Autodesk Inventor part; units mm, degrees
ref_plane "Work Plane1" through (29, 0, 0) normal (0, -1, 0) x (1, 0, 0)
ref_plane "YZ Plane" through (0, 0, 0) normal (1, 0, 0) x (0, 1, 0)
ref_plane "XZ Plane" through (0, 0, 0) normal (0, 1, 0) x (-1, 0, 0)
sketch "Skizze1" plane through (0, 0, 0) normal (0, 0, 1) x (1, 0, 0)
  line L0 (-1.1667, 0) -> (20, 0)
  line L1 (20, 0) -> (20, 2.5)
  line L2 (20, 2.5) -> (2, 2.5)
  line L3 (2, 2.5) -> (1.5091, 2.5)
  line L4 (1.5091, 2.5) -> (0, 2.5)
  line L5 (0, 2.5) -> (0, 4.25)
  line L6 (0, 4.25) -> (-5, 4.25)
  line L7 (-5, 4.25) -> (-5, 2.3094)
  line L8 (-5, 2.3094) -> (-2.5, 2.3094)
  line L9 (-2.5, 2.3094) -> (-1.1667, 0)
  line L10 (-10, 0) -> (25, 0)
  line L11 (0, -0.85) -> (0, 5.1)
  line L12 (2, 2.5) -> (0, 2.5) construction
  dimension "d1" = 18
  dimension "d2" = 0.4909
  dimension "d3" = 5
  dimension "d4" = 2.5
  dimension "d5" = 60
  dimension "d6" = 5
  dimension "d7" = 5
  dimension "d8" = 4.6188
  dimension "d9" = 8.5
  dimension "d26" = 20
revolve "Körper" add sketch "Skizze1" angle 360 about axis through (-1.1667, 0, 0) along (1, 0, 0)
sketch "Skizze2" plane through (-5, 0, 0) normal (-1, 0, 0) x (0, 0, 1)
  circle A0 centre (0, 0) radius 2.3094
  line L0 (0, -5.95) -> (0, 5.95)
  line L1 (-5.95, 0) -> (5.95, 0)
  line L2 (2.3094, 0) -> (1.1547, -2)
  line L3 (1.1547, -2) -> (-1.1547, -2)
  line L4 (-1.1547, -2) -> (-2.3094, 0)
  line L5 (-2.3094, 0) -> (-1.1547, 2)
  line L6 (-1.1547, 2) -> (1.1547, 2)
  line L7 (1.1547, 2) -> (2.3094, 0)
extrude "Loch" add sketch "Skizze2" against normal up to next contours L7 A0 | A0 L2 | L6 L0 A0 | A0 L0 L3 | L0 L6 A0 | A0 L3 L0 | L4 A0 | A0 L5
fillet "Rundung1" radius 0.5 1 edges at (-5, -4.25, 0)
thread "Gewinde"
chamfer "Fase1" distance 0.4908 distance2 0.4908 1 edges at (20, -2.5, 0) measured on face at (20, -0.7379, -0.3873)
ref_plane "Work Plane1" through (29, 0, 0) normal (0, -1, 0) x (1, 0, 0)
fillet "Fillet2" radius 0.1 1 edges at (0, -2.5, 0)
sketch "Skizze4" plane through (0, 0, 0) normal (0, 1, 0) x (-1, 0, 0)
  line L0 (-19.5092, 2.5) -> (-19.5092, -2.5)
  line L1 (-0.1, -2.5) -> (-0.1, 2.5)
  line L2 (-0.1, 2.5) -> (-19.5092, 2.5)
  line L3 (-6.74, 2.5) -> (-6, 2.5)
  line L4 (-6, 2.5) -> (-6, 1.6)
  line L5 (-6, 1.6) -> (-6.74, 1.6)
  line L6 (-6.74, 1.6) -> (-6.74, 2.5)
  line L7 (0, 4.25) -> (0, -4.25)
  line L8 (10, 0) -> (-25, 0)
  point P0 (0, 0)
  dimension "d31" = 6
  dimension "d32" = 3.2
  dimension "d33" = 0.74
revolve "Umdrehung2" cut sketch "Skizze4" angle 360 about axis through (-10, 0, 0) along (1, 0, 0) contours L2 L4 L5 L6
equation "\"d30\" = R"
equation "\"d17\" = RR"
equation "\"d13\" = GEL"
equation "\"d15\" = -0.5 * SPD + 0.5 * GD"
equation "\"d16\" = GUL"
equation "\"d1\" = GEL"
equation "\"d3\" = KOH"
equation "\"d4\" = INTI"
equation "\"d6\" = GD"
equation "\"d7\" = BDM"
equation "\"d8\" = 1.1547 * SW"
equation "\"d9\" = KOD"
equation "\"d26\" = NLG"
equation "\"GD\" = 5"
equation "\"NLG\" = 20"
equation "\"GEL\" = 18"
equation "\"KOD\" = 8.5"
equation "\"KOH\" = 5"
equation "\"INTI\" = 2.5"
equation "\"GAL\" = 0.61345 * PTC"
equation "\"GUL\" = 0.61345 * PTC"
equation "\"BDM\" = NND"
equation "\"SW\" = 4"
equation "\"RR\" = 0.5"
equation "\"SPD\" = NND - 1.2269 * PTC"
equation "\"R\" = 0.1"
equation "\"TOA\" = 30deg"
equation "\"GD1\" = THREADDIA - 1.2269 * PTC"
equation "\"THREADDIA\" = 5"
equation "\"FAWI\" = 45deg"
equation "\"PTC\" = 0.8"
equation "\"NND\" = 5"
equation "\"E0\" = 1.155 * SW"
properties part number "ISO 4762 - M5 x 20" material "EdelStahl - 440C"
Source: CAD feature listing. Evaluate the final solid. Frame: model axes, mm. A direction names the side the tool comes from. Coordinates: 2 decimals unless noted, no trailing zeros. Write each loop counter-clockwise with the first axis right and the second up, starting at its lowest first coordinate (ties: lowest second). Pieces come first, ordered by that corner, then holes. Notation, with made-up numbers: (32, -19) -> (46, -19) arc R33 cw to (46, 11) -> close; hole circle Ø10 at (37.25, -29.75). An arc over 180 degrees is marked (long way). Return JSON: item names as keys, results as strings. Group by question number.
1) Ray query, line 1 along Z through (x, y) = (16.25, -1.5); line 2 along Z through (x, y) = (-2.75, 1.75); line 3 along X through (y, z) = (1.75, -0.25). Return the intervals inside material, ascending.
2) Section query A-A, the plane x = -3. Return loops of the section in (y, z).
3) Mould query, pull axis X, two halves, no side actions, for faces 1 (the face through (13.04, -0.54, 2.44)), 2 (the face through (6.38, 0.97, -1.27)), 3 (the face through (0, 2, 2)), 4 (the face through (6.74, 0, 2)). Classes: +X half, -X half, draft (parallel to the pull), parting line (faces both ways), or undercut.
4) Set-up query: faces 5 (the face through (3.01, -0.54, 2.44)), 6 (the face through (-4, 2, 0)), 7 (the face through (6, 0, 2)). Return all of +Z, -Z, +X, -X, +Y, -Y with unobstructed straight access to the full face (end or side cutting, diameter ignored); none if empty.
5) Contact query for flat-ended pins moving along their axis: P1, Ø2, axis at y = -0.5, z = 3, coming from the +X side; P2, Ø4, axis at x = 8.5, y = -0.5, coming from the +Z side; P3, Ø0.7, axis at x = -3.5, z = -0.5, coming from the -Y side. Output: stop coordinate, or through.
6) Section query B-B, the plane x = 17.75. Return loops of the section in (y, z).
From the geometry:
{
 "1": {"line 1": "-2 to 2", "line 2": "-3.87 to -1.3, 1.3 to 3.87", "line 3": "-2.19 to 6, 6.74 to 20"},
 "2": {"outline": "circle Ø8.5 at (0, 0); hole (-2, -1.15) -> (0, -2.31) -> (2, -1.15) -> (2, 1.15) -> (0, 2.31) -> (-2, 1.15) -> close"},
 "3": {"face 1": "draft", "face 2": "undercut", "face 3": "+X half", "face 4": "undercut"},
 "4": {"face 5": "+X", "face 6": "-X", "face 7": "none"},
 "5": {"P1": "x = 19.97", "P2": "z = 2.5", "P3": "y = -4.25"},
 "6": {"outline": "circle Ø5 at (0, 0)"}
}
